The listing builds one solid part. Answer for the finished solid, in the listing's coordinates (mm). Face numbers are marked on the shaded views. Round coordinates to 2 decimals unless told otherwise and drop trailing zeros. Order: outer loops, then holes, each group sorted by start corner. A loop starts at its lowest first (then second) coordinate and runs counter-clockwise, first axis right, second up. Notation, with made-up numbers: (-30.75, -11) -> (10.25, -11) arc R24 cw to (10.25, 3) -> close; hole circle Ø8 at (42, -2). An arc over 180 degrees is marked (long way). Return JSON: item names as keys, results as strings. Group by question number.
(1) Determine the mould class of the marked faces 1 and 2 for opening direction Z: +Z half, -Z half, draft (parallel to the pull), parting line (faces both ways), or undercut.
(2) The part is cut by section A-A (z = 2). Determine the outline of the cut face in (x, y).
(3) The part is cut by section C-C (y = -65). Determine the outline of the cut face in (x, z), plus the area to 3 significant figures.
(4) Each of these flat-tipped pins is pushed along its axis until it touches: pin 1 (5 mm diameter, centred on x = 184.73, y = -21, fed in from -Z); pin 2 (3.5 mm diameter, centred on x = 28, y = -14, fed in from +Z); pin 3 (3 mm diameter, centred on x = 121, z = 8.5, fed in from -Y); pin 4 (4 mm diameter, centred on y = -133, z = 6.5, fed in from +X). Where does it stop, or does it pass through?
(5) The part is cut by section B-B (x = 177.5). Determine the outline of the cut face in (y, z), plus the area to 3 significant figures.
(6) Consider line 1 (Y direction, x = 27.5, z = 7); line 2 (Y direction, x = 27.5, z = 11.8); line 3 (X direction, y = -15, z = 10.6). Determine where each line is inside the solid, lowest interval first. Write a range as [from, to].
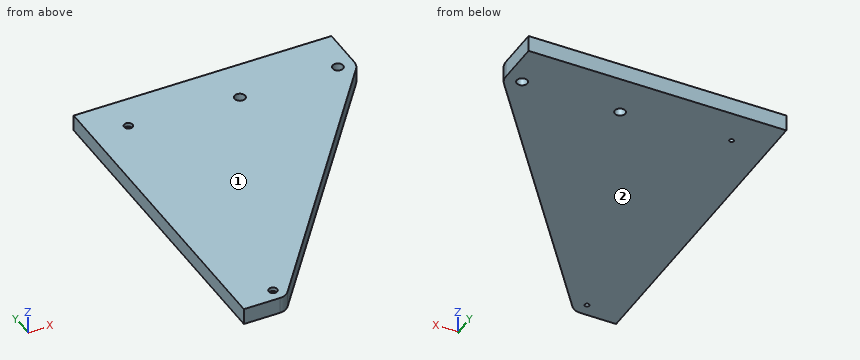
Autodesk Inventor part; units mm, degrees
ref_plane "YZ Plane" through (0, 0, 0) normal (1, 0, 0) x (0, 1, 0)
ref_plane "XZ Plane" through (0, 0, 0) normal (0, 1, 0) x (-1, 0, 0)
ref_plane "XY Plane" through (0, 0, 0) normal (0, 0, 1) x (1, 0, 0)
ref_plane "Work Plane1" through (0, 142.0555, 0) normal (0, 0, 1) x (1, 0, 0)
sketch "Sketch1" plane through (0, 142.0555, 0) normal (0, 0, 1) x (1, 0, 0)
  line L0 (450, -129.5555) -> (450, -142.0555)
  line L1 (0, -129.5555) -> (450, -129.5555)
  line L2 (0, -142.0555) -> (0, -129.5555)
  line L3 (450, -142.0555) -> (0, -142.0555)
  circle A0 centre (109.7339, -163.0555) radius 4.05
  circle A1 centre (184.7339, -163.0555) radius 4.05
  line L4 (92.2339, -147.0555) -> (92.2339, -142.0555)
  arc A2 (97.2339, -152.0555) -> (92.2339, -147.0555) centre (92.2339, -152.0555) ccw
  line L5 (97.2339, -152.0555) -> (97.2339, -163.0555)
  arc A3 (97.2339, -163.0555) -> (122.2339, -163.0555) centre (109.7339, -163.0555) ccw
  line L6 (122.2339, -163.0555) -> (122.2339, -152.0555)
  arc A4 (127.2339, -147.0555) -> (122.2339, -152.0555) centre (127.2339, -152.0555) ccw
  line L7 (127.2339, -147.0555) -> (167.2339, -147.0555)
  arc A5 (172.2339, -152.0555) -> (167.2339, -147.0555) centre (167.2339, -152.0555) ccw
  line L8 (172.2339, -152.0555) -> (172.2339, -163.0555)
  arc A6 (172.2339, -163.0555) -> (197.2339, -163.0555) centre (184.7339, -163.0555) ccw
  line L9 (197.2339, -163.0555) -> (197.2339, -152.0555)
  arc A7 (202.2339, -147.0555) -> (197.2339, -152.0555) centre (202.2339, -152.0555) ccw
  line L10 (202.2339, -142.0555) -> (202.2339, -147.0555)
  line L11 (92.2339, -142.0555) -> (202.2339, -142.0555)
  line L12 (0, -129.5555) -> (0, -379.5555)
  line L13 (0, -379.5555) -> (27.5, -379.5555)
  line L14 (35.3974, -375.6899) -> (194.6057, -170.7235)
  line L15 (197.2339, -163.0555) -> (197.2339, -129.5555)
  line L16 (0, -129.5555) -> (197.2339, -129.5555)
  arc A8 (194.6057, -170.7235) -> (197.2339, -163.0555) centre (184.7339, -163.0555) ccw
  arc A9 (27.5, -379.5555) -> (35.3974, -375.6899) centre (27.5, -369.5555) ccw
  dimension "d2" = 250
  dimension "d5" = 20
  dimension "d6" = 27.5
extrude "Extrusion1" add sketch "Sketch1" along normal blind 12.5 contours L15 L3 L2 L1 | L15 L9 A6 L8 A5 L7 A4 L6 A3 L5 A2 L4 L3 | L3 L4 A2 L5 A3 L6 A4 L7 A5 L8 A6 L14 A9 L13 L12
sketch "Sketch2" plane through (0, 142.0555, 0) normal (0, 0, -1) x (-1, 0, 0)
  circle A0 centre (-27.5, -369.5555) radius 1.55
  circle A1 centre (-27.5, -157.0555) radius 1.55
  point P0 (0, -142.0555)
extrude "Extrusion2" cut sketch "Sketch2" against normal through all
sketch "Sketch3" plane through (0, 142.0555, 12.5) normal (0, 0, 1) x (1, 0, 0)
  circle A0 centre (27.5, -157.0555) radius 1.55
  arc A1 (27.5, -379.5555) -> (35.3974, -375.6899) centre (27.5, -369.5555) ccw
  point P0 (0, -142.0555)
hole "Hole1" at (27.5, -15, 12.5) at (27.5, -227.5, 12.5) direction (0, 0, -1) diameter 3.4036 end through all counterbore diameter 6.5024 counterbore depth 2.9972
properties part number "side support"
Answer below:
{
 "1": {"face 1": "+Z half", "face 2": "-Z half"},
 "2": {"outline": "(0, -237.5) -> (27.5, -237.5) arc R10 ccw to (35.4, -233.63) -> (194.61, -28.67) arc R12.5 ccw to (197.23, -21) -> (197.23, 12.5) -> (0, 12.5) -> close; hole circle Ø3.4 at (27.5, -227.5); hole circle Ø3.4 at (27.5, -15); hole circle Ø8.1 at (109.73, -21); hole circle Ø8.1 at (184.73, -21)"},
 "3": {"outline": "(0, 0) -> (166.38, 0) -> (166.38, 12.5) -> (0, 12.5) -> close", "area": "2,080 mm²"},
 "4": {"pin 1": "passes through", "pin 2": "stops at z = 9.5", "pin 3": "stops at y = -125.36", "pin 4": "stops at x = 115.12"},
 "5": {"outline": "(-50.69, 0) -> (12.5, 0) -> (12.5, 12.5) -> (-50.69, 12.5) -> close", "area": "790 mm²"},
 "6": {"line 1": "y = [-237.5, -229.2], [-225.8, -16.7], [-13.3, 12.5]", "line 2": "y = [-237.5, -230.75], [-224.25, -18.25], [-11.75, 12.5]", "line 3": "x = [0, 24.25], [30.75, 197.23]"}
}
